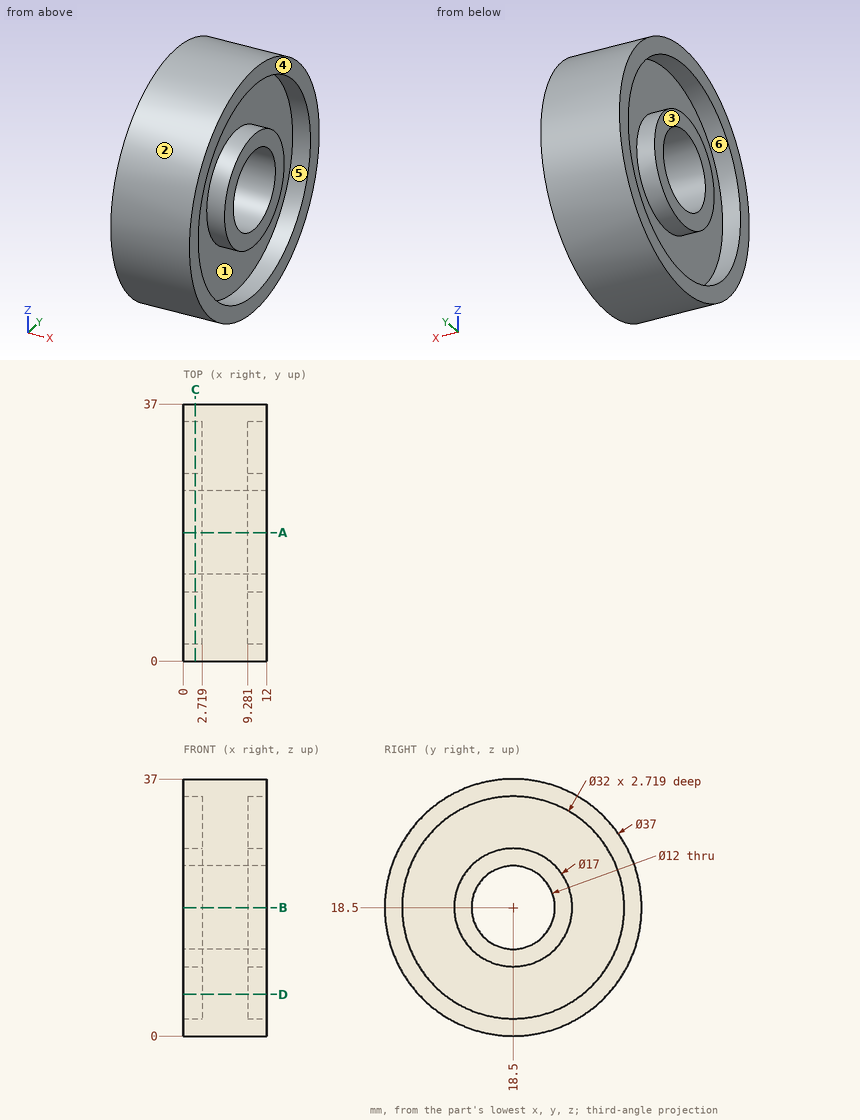
Input: dimensioned drawing with shaded views. Units: mm. Origin: part minimum x, y, z. A direction names the side the tool comes from. Coordinates: 2 decimals unless noted, no trailing zeros. Order: outer loops, then holes, each group sorted by start corner. A loop starts at its lowest first (then second) coordinate and runs counter-clockwise, first axis right, second up. Notation, with made-up numbers: (30, -36) -> (39, -36) arc R19 ccw to (39, -15) -> close; hole circle Ø4 at (68.5, 4.25). An arc over 180 degrees is marked (long way). Answer in a Markdown table with one row per item.
Item 1: Section A-A on y = 18.5. Output: boundary loops of the cut face in (x, z).
Return value:
| item | result |
|---|---|
| outline | (0, 0) -> (12, 0) -> (12, 2.5) -> (9.28, 2.5) -> (9.28, 10) -> (12, 10) -> (12, 12.5) -> (0, 12.5) -> (0, 10) -> (2.72, 10) -> (2.72, 2.5) -> (0, 2.5) -> close; (0, 24.5) -> (12, 24.5) -> (12, 27) -> (9.28, 27) -> (9.28, 34.5) -> (12, 34.5) -> (12, 37) -> (0, 37) -> (0, 34.5) -> (2.72, 34.5) -> (2.72, 27) -> (0, 27) -> close |
Item 2: Ray query, L1, parallel to Y at x = 10, z = 18.5; L2, parallel to Y at x = 9.75, z = 20.5 (1 decimal); L3, parallel to Y at x = 4, z = 18.5. Return the intervals inside material, ascending.
Return value:
| item | result |
|---|---|
| L1 | y = 0 to 2.5, 10 to 12.5, 24.5 to 27, 34.5 to 37 |
| L2 | y = 0.1 to 2.6, 10.2 to 12.8, 24.2 to 26.8, 34.4 to 36.9 |
| L3 | y = 0 to 12.5, 24.5 to 37 |
Item 3: Access query for the marked faces 4, 5 and 6. Directions: +Z, -Z, +X, -X, +Y, -Y. A direction counts if a zero-diameter tool reaches every point of the face in a straight line with its end or side. Return the directions, or none.
Return value:
| item | result |
|---|---|
| face 4 | +Z, -Z, +X, +Y, -Y |
| face 5 | +X |
| face 6 | -X |
Item 4: Contact query for flat-ended pins moving along their axis: P1, Ø4, axis at x = 3.5, z = 13.5, coming from the +Y side (3 decimals); P2, Ø4, axis at x = 3.5, z = 10.5, coming from the -Y side; P3, Ø6, axis at x = 6.5, z = 22.5, coming from the +Y side. Output: stop coordinate, or through.
Return value:
| item | result |
|---|---|
| P1 | stops at y = 36.755 |
| P2 | stops at y = 1 |
| P3 | stops at y = 36.97 |
Item 5: Section C-C on x = 1.75. Output: boundary loops of the cut face in (y, z).
Return value:
| item | result |
|---|---|
| outline | circle Ø37 at (18.5, 18.5); circle Ø17 at (18.5, 18.5); hole circle Ø32 at (18.5, 18.5); hole circle Ø12 at (18.5, 18.5) |
Item 6: Section D-D on z = 6. Output: boundary loops of the cut face in (x, y), plus the area to 3 significant figures.
Return value:
| item | result |
|---|---|
| outline | (0, 4.86) -> (12, 4.86) -> (12, 8.51) -> (9.28, 8.51) -> (9.28, 28.49) -> (12, 28.49) -> (12, 32.14) -> (0, 32.14) -> (0, 28.49) -> (2.72, 28.49) -> (2.72, 8.51) -> (0, 8.51) -> close |
| area | 219 mm² |
Item 7: Draft query along Z for the marked faces 1, 2 and 3. Return one class per face: released by +Z, released by -Z, zero draft, split by the parting line, or undercut.
Return value:
| item | result |
|---|---|
| face 1 | undercut |
| face 2 | split by the parting line |
| face 3 | zero draft |
